```python
from build123d import *

# Parameters (mm, degrees)
SKETCH1_R             = 1
BOSS_EXTRUDE1_DEPTH   = 5
BOSS_EXTRUDE1_2_DEPTH = 5
BOSS_EXTRUDE1_3_DEPTH = 5
BOSS_EXTRUDE1_4_DEPTH = 5
SKETCH2_R             = 3
BOSS_EXTRUDE2_DEPTH   = 5
SKETCH3_R             = 1
CUT_EXTRUDE2_DEPTH    = 10


with BuildPart() as part:
    # Sketch1 → Boss-Extrude1 (new body)
    with BuildSketch(Plane.XY):
        with Locations((8, 1)):
            Circle(SKETCH1_R)
    extrude(amount=BOSS_EXTRUDE1_DEPTH)



with BuildPart() as body_2:
    # Sketch1 → Boss-Extrude1 2 (new body)
    with BuildSketch(Plane.XY):
        with Locations((8, 8)):
            Circle(SKETCH1_R)
    extrude(amount=BOSS_EXTRUDE1_2_DEPTH)


with BuildPart() as body_3:
    # Sketch1 → Boss-Extrude1 3 (new body)
    with BuildSketch(Plane.XY):
        with Locations((1, 8)):
            Circle(SKETCH1_R)
    extrude(amount=BOSS_EXTRUDE1_3_DEPTH)


with BuildPart() as body_4:
    # Sketch1 → Boss-Extrude1 4 (new body)
    with BuildSketch(Plane.XY):
        with Locations((1, 1)):
            Circle(SKETCH1_R)
    extrude(amount=BOSS_EXTRUDE1_4_DEPTH)


with BuildPart() as part_1:
    add(part.part)

    add(body_2.part)  # Boss-Extrude2 merges body 2

    add(body_3.part)  # Boss-Extrude2 merges body 3

    add(body_4.part)  # Boss-Extrude2 merges body 4
    # Sketch2 → Boss-Extrude2 (add)
    with BuildSketch(Plane.XY.offset(5)):
        with BuildLine():
            Line((4, -5), (5, -5))
            ThreePointArc((5, -5), (9.949747468, -2.949747468), (12, 2))
            Line((12, 2), (12, 108))
            ThreePointArc((12, 108), (9.949747468, 112.949747468), (5, 115))
            Line((5, 115), (4, 115))
            ThreePointArc((4, 115), (-0.949747468, 112.949747468), (-3, 108))
            Line((-3, 108), (-3, 2))
            ThreePointArc((-3, 2), (-0.949747468, -2.949747468), (4, -5))
        make_face()
        with Locations((4.5, 108)):
            Circle(SKETCH2_R, mode=Mode.SUBTRACT)
    extrude(amount=BOSS_EXTRUDE2_DEPTH)

    # Sketch3 → Cut-Extrude2 (cut)
    with BuildSketch(Plane(origin=(0, 0, 0), x_dir=(-1, 0, 0), z_dir=(0, 0, -1))):
        with Locations((-8, 8)):
            Circle(SKETCH3_R)
        with Locations((-1, 8)):
            Circle(SKETCH3_R)
        with Locations((-1, 1)):
            Circle(SKETCH3_R)
        with Locations((-8, 1)):
            Circle(SKETCH3_R)
    extrude(amount=-CUT_EXTRUDE2_DEPTH, mode=Mode.SUBTRACT)


solid = part_1.part
```
Geometry check sheet. Reference: the model listing, model coordinates, mm. Coordinates: 2 decimals unless noted, no trailing zeros. Order: outer loops, then holes, each group sorted by start corner. A loop starts at its lowest first (then second) coordinate and runs counter-clockwise, first axis right, second up.
Item 1: Depth check by flat-ended pin: pin 1 (1 mm diameter, centred on x = 8, z = 5.5, fed in from +Y). Enter the tip coordinate at first touch or a pass-through.
Item 2: Section check B-B (z = 6.4). Enter the section's corners in (x, y).
Item 3: Scan lines: line 1 along Y through (x, z) = (1.25, 6.65); line 2 along Y through (x, z) = (4.5, 6.7); line 3 along Y through (x, z) = (1, 6.8). Record each from-to range of solid material in increasing order.
Item 4: Section check A-A (y = 8). Enter the section's corners in (x, z).
Item 5: Mould release check, pull along X, two halves, no side actions. Record for faces 1 (the cylindrical face through (3.85, 105.07, 7.46)), 2 (the cylindrical face through (-1, -2.9, 7.5)), 3 (the flat face through (4, 56, 10)): released by +X, released by -X, zero draft, split by the parting line, or undercut.
Check sheet entries:
1. pin 1: stops at y = 114.54
2. outline: (-3, 2) arc R7 ccw to (4, -5) - (5, -5) arc R7 ccw to (12, 2) - (12, 108) arc R7 ccw to (5, 115) - (4, 115) arc R7 ccw to (-3, 108) - close; hole circle Ø2 at (1, 1); hole circle Ø2 at (1, 8); hole circle Ø6 at (4.5, 108); hole circle Ø2 at (8, 1); hole circle Ø2 at (8, 8)
3. line 1: y = -4.44 to 0.03, 1.97 to 7.03, 8.97 to 114.44
3. line 2: y = -5 to 105, 111 to 115
3. line 3: y = -4.32 to 0, 2 to 7, 9 to 114.32
4. outline: (-3, 5) - (0, 5) - (0, 10) - (-3, 10) - close; (2, 5) - (7, 5) - (7, 10) - (2, 10) - close; (9, 5) - (12, 5) - (12, 10) - (9, 10) - close
5. face 1: undercut
5. face 2: released by -X
5. face 3: zero draft
